from build123d import *

# Parameters (mm, degrees)
F0_W      = 35
F0_H      = 10
F1_DEPTH  = 3
F2_R      = 1.5
F4_DEPTH  = 3
F6_DEPTH  = 6
F7_R      = 1
F8_R      = 1.25
F10_DEPTH = 3
F9_R      = 1.25
F11_DEPTH = 3


with BuildPart() as f1:
    # F0 (on Top) → F1 (new body)
    with BuildSketch(Plane.XY):
        with Locations((11.178067, 1.255235)):
            Rectangle(F0_W, F0_H)
    extrude(amount=F1_DEPTH)

    # F2
    f2_edges = [f1.edges().sort_by_distance(p)[0] for p in [
        (-6.321933, -3.744765, 1.5),
        (-6.321933, 6.255235, 1.5),
        (28.678067, -3.744765, 1.5),
        (28.678067, 6.255235, 1.5),
    ]]
    fillet(f2_edges, radius=F2_R)

    # F3 (on face) → F4 (join)
    with BuildSketch(Plane.XY.offset(3)):
        with BuildLine():
            ThreePointArc((11.178067, -3.744765), (14.713601, -2.280299), (16.178067, 1.255235))
            ThreePointArc((16.178067, 1.255235), (14.713601, 4.790769), (11.178067, 6.255235))
            ThreePointArc((11.178067, 6.255235), (6.178067, 1.255235), (11.178067, -3.744765))
        make_face()
    extrude(amount=F4_DEPTH)

    # F5 (on face) → F6 (cut)
    with BuildSketch(Plane.XY.offset(6)):
        with BuildLine():
            ThreePointArc((13.428067, 1.255235), (12.545025, 3.042391), (10.589023, 3.426762))
            ThreePointArc((10.589023, 3.426762), (9.006541, 0.666191), (11.767111, -0.916291))
            ThreePointArc((11.767111, -0.916291), (12.965222, -0.111723), (13.428067, 1.255235))
        make_face()
        with BuildLine():
            Line((13.966953, 4.343053), (10.589023, 3.426762))
            ThreePointArc((10.589023, 3.426762), (12.545025, 3.042391), (13.428067, 1.255235))
            ThreePointArc((13.428067, 1.255235), (12.965222, -0.111723), (11.767111, -0.916291))
            Line((11.767111, -0.916291), (15.145041, 0))
            Line((15.145041, 0), (13.966953, 4.343053))
        make_face()
        with BuildLine():
            Line((10.589023, 3.426762), (7.211093, 2.51047))
            Line((7.211093, 2.51047), (8.389181, -1.832582))
            Line((8.389181, -1.832582), (11.767111, -0.916291))
            ThreePointArc((11.767111, -0.916291), (9.006541, 0.666191), (10.589023, 3.426762))
        make_face()
    extrude(amount=-F6_DEPTH, mode=Mode.SUBTRACT)

    # F7
    f7_edges = [f1.edges().sort_by_distance(p)[0] for p in [
        (7.211093, 2.51047, 3),
        (8.389181, -1.832582, 3),
        (15.145041, 0, 3),
        (13.966953, 4.343053, 3),
    ]]
    fillet(f7_edges, radius=F7_R)

    # F8 (on face) → F10 (cut)
    with BuildSketch(Plane.XY.offset(3)):
        with Locations((-3.321933, 1.255235)):
            Circle(F8_R)
    extrude(amount=-F10_DEPTH, mode=Mode.SUBTRACT)

    # F9 (on face) → F11 (cut)
    with BuildSketch(Plane.XY.offset(3)):
        with Locations((25.678067, 1.255235)):
            Circle(F9_R)
    extrude(amount=-F11_DEPTH, mode=Mode.SUBTRACT)


solid = f1.part
Geometry: final body of the model. Coordinates: model frame, mm. A direction names the side the tool comes from. Coordinates: 2 decimals unless noted, no trailing zeros. Loops run counter-clockwise (first coordinate to the right, second up) from the corner with the lowest first, then second, coordinate; pieces in that order, holes last. Notation, with made-up numbers: M -38.75,1.5 L 5.25,1.5 A15 cw 5.25,12.5 Z; hole C 7.25,72 d7. An arc over 180 degrees is marked long. One line per item, written item: value. Start each with the question number.
1) Draft query along X for faces 1 (the flat face through (-6.322, 1, 1)), 2 (the cylindrical face through (-2.745, 0.146, 1.521)), 3 (the flat face through (0, 1, 3)). Return one class per face: released by +X, released by -X, zero draft, split by the parting line, or undercut.
2) Cut plane C-C (x = 26.5). Return loops of the section in (y, z), then the cut area to 3 significant figures.
3) Pin query (flat end, axial travel): P1, Ø1, axis at x = -0.5, y = -0.5, coming from the +Z side; P2, Ø2, axis at x = 25.68, y = 1.26, coming from the +Z side. Return the tip coordinate at first contact, or that it passes through.
4) Reachability of faces 4 (the flat face through (28.678, 1, 1)), 5 (the flat face through (11.733, -0.925, 3.042)) from +Z, -Z, +X, -X, +Y, -Y: full face, straight path, thin tool, end or side. Return the list, or none.
5) Cut plane B-B (z = 1.6). Return loops of the section in (x, y), then the cut area to 3 significant figures.
6) Material intervals for L1, parallel to X at y = 1.5, z = 0.55; L2, parallel to Z at x = 2, y = 2.5; L3, parallel to Y at x = 11, z = 2, sorted ascending. Write a range as from..to.
7) Cut plane A-A (z = 3.7). Return loops of the section in (x, y).
8) Cut plane D-D (y = 3.75). Return loops of the section in (x, z).
Evaluation:
1. face 1: released by -X
1. face 2: undercut
1. face 3: zero draft
2. outline: M -3.74,0 L 0.31,0 L 0.31,3 L -3.74,3 Z; M 2.2,0 L 6.26,0 L 6.26,3 L 2.2,3 Z
2. area: 24.3 mm^2
3. P1: z = 3
3. P2: through
4. face 4: +Z, -Z, +X, +Y, -Y
4. face 5: +Z, -Z
5. outline: M -6.32,-2.24 A1.5 ccw -4.82,-3.74 L 27.18,-3.74 A1.5 ccw 28.68,-2.24 L 28.68,4.76 A1.5 ccw 27.18,6.26 L -4.82,6.26 A1.5 ccw -6.32,4.76 Z; hole C -3.32,1.26 d2.5; hole M 7.47,1.55 L 8.13,-0.87 A1 ccw 9.35,-1.57 L 14.18,-0.26 A1 ccw 14.88,0.97 L 14.23,3.38 A1 ccw 13,4.08 L 10.59,3.43 L 8.18,2.77 A1 ccw Z; hole C 25.68,1.26 d2.5
5. area: 308 mm^2
6. L1: -6.32..-4.55, -2.1..7.49, 14.74..24.45, 26.9..28.68
6. L2: 0..3
6. L3: -3.74..-1.12, 3.54..6.26
7. outline: C 11.18,1.26 d10; hole M 7.47,1.55 L 8.13,-0.87 A1 ccw 9.35,-1.57 L 14.18,-0.26 A1 ccw 14.88,0.97 L 14.23,3.38 A1 ccw 13,4.08 L 10.59,3.43 L 8.18,2.77 A1 ccw Z
8. outline: M -6.32,0 L 11.78,0 L 11.78,6 L 6.84,6 L 6.84,3 L -6.32,3 Z; M 14.04,0 L 28.68,0 L 28.68,3 L 15.51,3 L 15.51,6 L 14.04,6 Z
